Autodesk Inventor part; units mm, degrees
ref_plane "YZ Plane" through (0, 0, 0) normal (1, 0, 0) x (0, 1, 0)
ref_plane "XZ Plane" through (0, 0, 0) normal (0, 1, 0) x (-1, 0, 0)
ref_plane "XY Plane" through (0, 0, 0) normal (0, 0, 1) x (1, 0, 0)
sketch "Эскиз1" plane through (0, 0, 0) normal (0, 0, 1) x (1, 0, 0)
  line L0 (0, 0) -> (39, 0)
  line L1 (39, 0) -> (39, 74)
  line L2 (39, 74) -> (0, 74)
  line L3 (0, 74) -> (0, 0)
  dimension "d0" = 39
  dimension "d1" = 74
extrude "Выдавливание1" add sketch "Эскиз1" along normal blind 5.5
sketch "Эскиз2" plane through (0, 0, 5.5) normal (0, 0, 1) x (1, 0, 0)
  line L0 (39, 0) -> (39, 74)
  line L1 (39, 10) -> (10, 10)
  line L2 (10, 10) -> (10, 64)
  line L3 (10, 64) -> (39, 64)
  line L4 (39, 64) -> (39, 10)
  line L5 (0, 0) -> (39, 0)
  line L6 (39, 74) -> (0, 74)
  point P0 (39, 64)
  dimension "d4" = 10
  dimension "d5" = 10
  dimension "d6" = 29
extrude "Выдавливание2" cut sketch "Эскиз2" against normal blind 13.5
sketch "Эскиз3" plane through (0, 0, 5.5) normal (0, 0, 1) x (1, 0, 0)
  circle A0 centre (13, 4.5) radius 1.25
  circle A1 centre (13, 69.5) radius 1.25
  line L0 (39, 0) -> (39, 10)
  line L1 (39, 64) -> (39, 74)
  line L2 (0, 0) -> (39, 0)
  line L3 (39, 74) -> (0, 74)
  dimension "d9" = 26
  dimension "d10" = 26
  dimension "d11" = 2.5
  dimension "d12" = 2.5
  dimension "d13" = 65
  dimension "d14" = 4.5
  dimension "d15" = 4.5
extrude "Выдавливание3" cut sketch "Эскиз3" against normal blind 4.5
fillet "Сопряжение1" radius 2 4 edges at (39, 0, 2.75) (39, 74, 2.75) (0, 0, 2.75) (0, 74, 2.75)
properties part number "s-10-5_Holder"
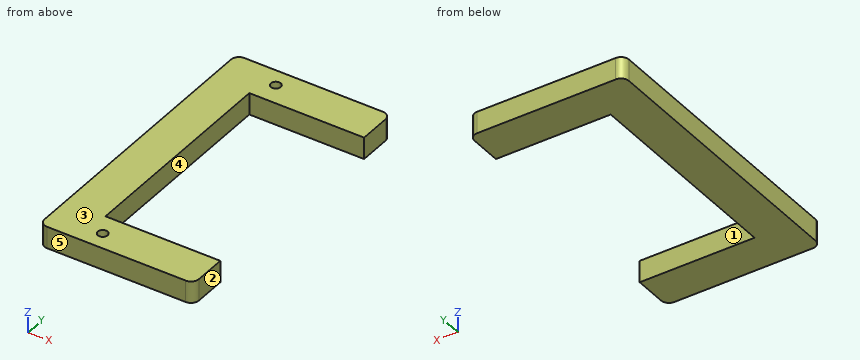
Verification items for the finished model (mm, model axes). Face numbers are marked on the shaded views. A direction names the side the tool comes from. Give positions to 0.01 mm unless a question says otherwise; leave off trailing zeros. Loops run counter-clockwise (first coordinate to the right, second up) from the corner with the lowest first, then second, coordinate; pieces in that order, holes last. Notation, with made-up numbers: M 64,59 L 86,59 A6 ccw 86,65 Z; hole C 8,60.25 d8. An arc over 180 degrees is marked long. Return JSON: item names as keys, results as strings.
1) Gauge pin test, flat ends, axial feed: P1, Ø3, axis at y = 43, z = 1.5, coming from the +X side; P2, Ø2, axis at x = 13, y = 69.5, coming from the +Z side. Record the tip position at first contact, or that the pin passes through.
Findings:
{"P1": "stops at x = 10", "P2": "stops at z = 1"}
2) Material ranges on L1, parallel to Y at x = 13, z = 2.7; L2, parallel to X at y = 69.5, z = 3.95; L3, parallel to Y at x = 19, z = 4.7, recorded low to high. Write a range as [from, to].
Findings:
{"L1": "y = [0, 3.25], [5.75, 10], [64, 68.25], [70.75, 74]", "L2": "x = [0, 11.75], [14.25, 39]", "L3": "y = [0, 10], [64, 74]"}
3) Section check D-D, the plane y = 29.5. Enter the section's corners in (x, z).
Findings:
{"outline": "M 0,0 L 10,0 L 10,5.5 L 0,5.5 Z"}
4) Section check A-A, the plane x = 15. Enter the section's corners in (y, z), and give its area (3 significant figures).
Findings:
{"outline": "M 0,0 L 10,0 L 10,5.5 L 0,5.5 Z; M 64,0 L 74,0 L 74,5.5 L 64,5.5 Z", "area": "110 mm2"}
5) Mould release check, pull along Y, two halves, no side actions. Record for the marked faces 3, 4 and 5: released by +Y, released by -Y, zero draft, split by the parting line, or undercut.
Findings:
{"face 3": "zero draft", "face 4": "undercut", "face 5": "released by -Y"}
6) Section check B-B, the plane z = 3.6. Enter the section's corners in (x, y), and give its area (3 significant figures).
Findings:
{"outline": "M 0,2 A2 ccw 2,0 L 37,0 A2 ccw 39,2 L 39,10 L 10,10 L 10,64 L 39,64 L 39,72 A2 ccw 37,74 L 2,74 A2 ccw 0,72 Z; hole C 13,4.5 d2.5; hole C 13,69.5 d2.5", "area": "1,310 mm2"}
7) Section check C-C, the plane y = 4.5. Enter the section's corners in (x, z), and give its area (3 significant figures).
Findings:
{"outline": "M 0,0 L 39,0 L 39,5.5 L 14.25,5.5 L 14.25,1 L 11.75,1 L 11.75,5.5 L 0,5.5 Z", "area": "203 mm2"}
8) Tool access check on the marked faces 1 and 2. Record the directions out of +Z, -Z, +X, -X, +Y, -Y that give a thin tool (end or side, any length) a straight path to the whole face; none if there is none.
Findings:
{"face 1": "+Z, -Z, +X", "face 2": "+Z, -Z, +X, +Y, -Y"}
